Input: part model. Units: mm. Frame: model coordinates. Round coordinates to 2 decimals unless told otherwise and drop trailing zeros. Order: outer loops, then holes, each group sorted by start corner. A loop starts at its lowest first (then second) coordinate and runs counter-clockwise, first axis right, second up. Notation, with made-up numbers: (80, 34) -> (122, 34) arc R20 cw to (122, 73) -> close; hole circle Ø5 at (72.25, 82). An arc over 180 degrees is marked (long way). Answer as CSV lines item,"result". Start each with the question number.
1) Section query B-B, the plane y = -2.5. Output: boundary loops of the cut face in (x, z), and give its area (3 significant figures).
2) Line query: L1, parallel to X at y = -1.7, z = 72.5; L2, parallel to X at y = -2.4, z = 46; L3, parallel to X at y = -0.85, z = 85.5. Output: solid intervals per line, ascending.
3) First-contact query: P1, Ø1.5, axis at y = -1, z = 25, coming from the +X side; P2, Ø8, axis at x = 70.5, z = 63, coming from the -Y side; P3, Ø1.5, axis at y = -1, z = 48.5, coming from the -X side; P4, Ø0.9, axis at x = 71, y = -2, coming from the +Z side. Flat tips, straight axial feed; report the tip coordinate or a pass-through.
4) Section query A-A, the plane z = 41.5. Output: boundary loops of the cut face in (x, y).
5) Section query C-C, the plane z = 55.5. Output: boundary loops of the cut face in (x, y).
6) Section query D-D, the plane x = 53. Output: boundary loops of the cut face in (y, z), and give its area (3 significant figures).
```python
from build123d import *

# Parameters (mm, degrees)
F1_DEPTH = 3


with BuildPart() as f1:
    # F0 (on Front) → F1 (new body)
    with BuildSketch(Plane.XZ):
        with BuildLine():
            Line((70, 0), (94.969561, 0))
            ThreePointArc((94.969561, 0), (89.308441, 32.298913), (73, 60.74716))
            Line((73, 60.74716), (73, 24.099964))
            Line((73, 24.099964), (70, 24.099964))
            Line((70, 24.099964), (70, 64.18113))
            ThreePointArc((70, 64.18113), (55.195862, 77.28282), (38, 87.035725))
            Line((38, 87.035725), (38, 34.923317))
            Line((38, 34.923317), (35, 34.923317))
            Line((35, 34.923317), (35, 88.284865))
            ThreePointArc((35, 88.284865), (19.269689, 92.994067), (2.963333, 94.923317))
            Line((2.963333, 94.923317), (2.963333, 34.923317))
            Line((2.963333, 34.923317), (0, 34.923317))
            Line((0, 34.923317), (0, 94.969561))
            ThreePointArc((0, 94.969561), (-16.239168, 93.570865), (-32, 89.41598))
            Line((-32, 89.41598), (-32, 34.923317))
            Line((-32, 34.923317), (-35, 34.923317))
            Line((-35, 34.923317), (-35, 88.284865))
            ThreePointArc((-35, 88.284865), (-52.026967, 79.45069), (-66.931372, 67.375136))
            Line((-66.931372, 67.375136), (-66.931372, 24.099964))
            Line((-66.931372, 24.099964), (-69.931372, 24.099964))
            Line((-69.931372, 24.099964), (-69.931372, 64.2559))
            ThreePointArc((-69.931372, 64.2559), (-88.488895, 34.480906), (-94.969561, 0))
            Line((-94.969561, 0), (-69.931372, 0))
            Line((-69.931372, 0), (-35, 0))
            Line((-35, 0), (0, 0))
            Line((0, 0), (35, 0))
            Line((35, 0), (70, 0))
        make_face()
    extrude(amount=F1_DEPTH)


solid = f1.part
```
Findings:
1,outline,"(-94.97, 0) -> (94.97, 0) arc R94.97 ccw to (73, 60.75) -> (73, 24.1) -> (70, 24.1) -> (70, 64.18) arc R94.97 ccw to (38, 87.04) -> (38, 34.92) -> (35, 34.92) -> (35, 88.28) arc R94.97 ccw to (2.96, 94.92) -> (2.96, 34.92) -> (0, 34.92) -> (0, 94.97) arc R94.97 ccw to (-32, 89.42) -> (-32, 34.92) -> (-35, 34.92) -> (-35, 88.28) arc R94.97 ccw to (-66.93, 67.38) -> (-66.93, 24.1) -> (-69.93, 24.1) -> (-69.93, 64.26) arc R94.97 ccw to start"
1,area,"13,400 mm^2"
2,L1,"x = -61.34 to -35, -32 to 0, 2.96 to 35, 38 to 61.34"
2,L2,"x = -83.09 to -69.93, -66.93 to -35, -32 to 0, 2.96 to 35, 38 to 70, 73 to 83.09"
2,L3,"x = -41.34 to -35, -32 to 0, 2.96 to 35, 38 to 41.34"
3,P1,"stops at x = 91.82"
3,P2,"stops at y = -3"
3,P3,"stops at x = -82.09"
3,P4,"stops at z = 24.1"
4,outline,"(-85.42, -3) -> (-69.93, -3) -> (-69.93, 0) -> (-85.42, 0) -> close; (-66.93, -3) -> (-35, -3) -> (-35, 0) -> (-66.93, 0) -> close; (-32, -3) -> (0, -3) -> (0, 0) -> (-32, 0) -> close; (2.96, -3) -> (35, -3) -> (35, 0) -> (2.96, 0) -> close; (38, -3) -> (70, -3) -> (70, 0) -> (38, 0) -> close; (73, -3) -> (85.42, -3) -> (85.42, 0) -> (73, 0) -> close"
5,outline,"(-77.06, -3) -> (-69.93, -3) -> (-69.93, 0) -> (-77.06, 0) -> close; (-66.93, -3) -> (-35, -3) -> (-35, 0) -> (-66.93, 0) -> close; (-32, -3) -> (0, -3) -> (0, 0) -> (-32, 0) -> close; (2.96, -3) -> (35, -3) -> (35, 0) -> (2.96, 0) -> close; (38, -3) -> (70, -3) -> (70, 0) -> (38, 0) -> close; (73, -3) -> (77.06, -3) -> (77.06, 0) -> (73, 0) -> close"
6,outline,"(-3, 0) -> (0, 0) -> (0, 78.8) -> (-3, 78.8) -> close"
6,area,"236 mm^2"
